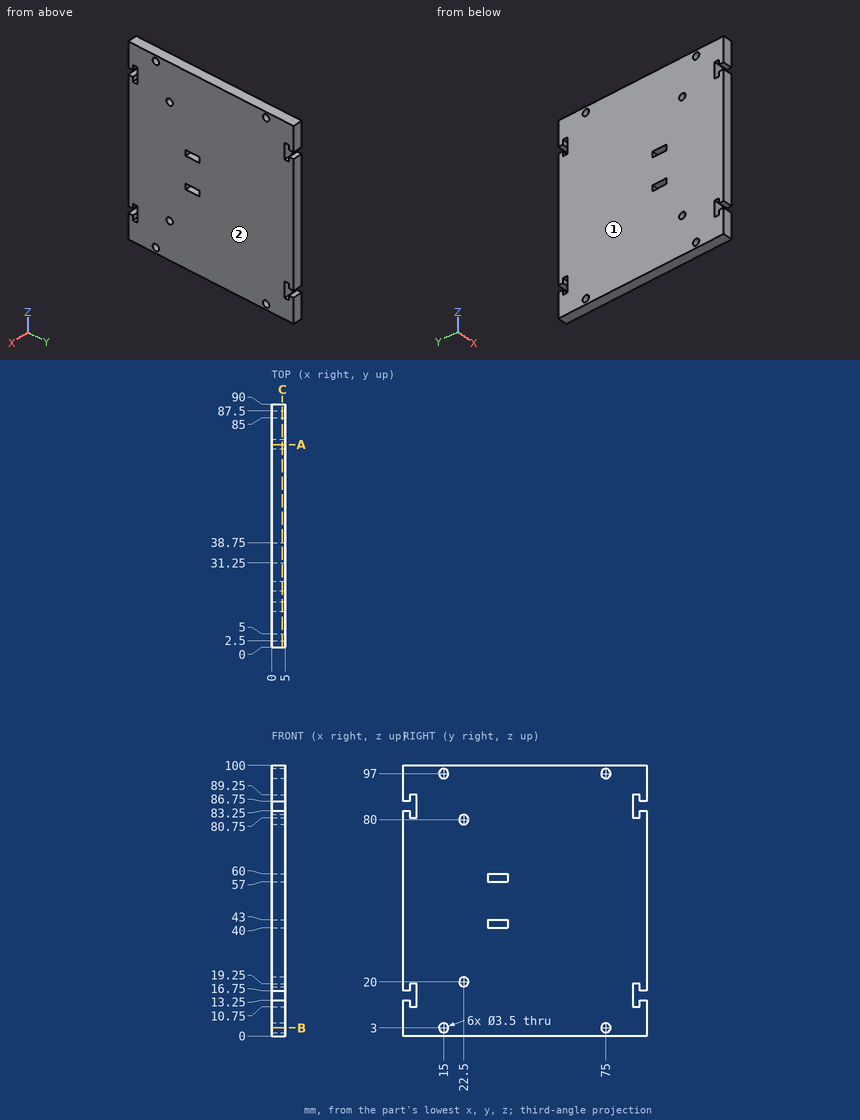
For this review, use the dimensioned drawing (mm, ordinates from the lowest corner) and the shaded views. Round coordinates to 2 decimals unless told otherwise and drop trailing zeros. Order: outer loops, then holes, each group sorted by start corner. A loop starts at its lowest first (then second) coordinate and runs counter-clockwise, first axis right, second up. Notation, with made-up numbers: M 2,75 L 51,75 A11 ccw 51,94 Z; hole C 77.5,33 d1. An arc over 180 degrees is marked long. Use a Markdown table: item, result.
1) Consider section C-C (x = 4.05). Give the number of separate pieces and of enclosed holes in the cut face, then the cut area to 3 significant figures.
Report:
| item | result |
|---|---|
| separate pieces | 1 |
| enclosed holes | 8 |
| area | 8,780 mm^2 |
2) Wall thickness on line 1 along Y through (x, z) = (3.6, 97); line 2 along Z through (x, y) = (3.7, 4.5); line 3 along Z through (x, y) = (1.2, 75): over which ranges is each line inside the solid? List them lowest first. Write a range as [from, to].
Report:
| item | result |
|---|---|
| line 1 | [0, 13.25], [16.75, 73.25], [76.75, 90] |
| line 2 | [0, 10.75], [19.25, 80.75], [89.25, 100] |
| line 3 | [0, 1.25], [4.75, 95.25], [98.75, 100] |
3) Consider section A-A (y = 75). Write out the cut boundary in (x, z).
Report:
| item | result |
|---|---|
| outline | M 0,0 L 5,0 L 5,1.25 L 0,1.25 Z; M 0,4.75 L 5,4.75 L 5,95.25 L 0,95.25 Z; M 0,98.75 L 5,98.75 L 5,100 L 0,100 Z |
4) Draft analysis for pull direction X (two halves, no side actions). For the marked faces 1 and 2, state which applies: released by +X, released by -X, zero draft, split by the parting line, or undercut.
Report:
| item | result |
|---|---|
| face 1 | released by -X |
| face 2 | released by +X |
5) Consider section B-B (z = 3). Write out the cut boundary in (x, y), then the cut area to 3 significant figures.
Report:
| item | result |
|---|---|
| outline | M 0,0 L 5,0 L 5,13.25 L 0,13.25 Z; M 0,16.75 L 5,16.75 L 5,73.25 L 0,73.25 Z; M 0,76.75 L 5,76.75 L 5,90 L 0,90 Z |
| area | 415 mm^2 |
6) Insertion check: pin 1 (2 mm diameter, centred on x = 3, z = 84.5, fed in from -Y); pin 2 (3 mm diameter, centred on y = 15, z = 3, fed in from +X). Each pin has a flat end and moves straight along its axis. Give the tip position at first contact, or say it passes through.
Report:
| item | result |
|---|---|
| pin 1 | y = 5 |
| pin 2 | through |
